Geometry: final body of the model. Coordinates: model frame, mm. A direction names the side the tool comes from. Give positions to 0.01 mm unless a question says otherwise; leave off trailing zeros.
1. Material intervals for line 1 along X through (y, z) = (-10.8, 421.85); line 2 along X through (y, z) = (11, 220) (3 decimals); line 3 along Y through (x, z) = (3, 393.5) (3 decimals), sorted ascending.
2. Access query for faces 1 (the face through (-2, -9.525, 332)), 2 (the face through (12.7, 0, 332)). Directions: +Z, -Z, +X, -X, +Y, -Y. A direction counts if a zero-diameter tool reaches every point of the face in a straight line with its end or side. Return the directions, or none.
3. First-contact query: P1, Ø12, axis at x = -1, y = -7.5, coming from the -Z side; P2, Ø4.5, axis at y = 2.38, z = 117.35, coming from the -X side (3 decimals); P3, Ø1, axis at y = -10, z = 199, coming from the -X side; P4, Ø4, axis at x = -2.38, z = 247.85, coming from the +Y side (3 decimals). Flat tips, straight axial feed; report the tip coordinate or a pass-through.
from build123d import *

# Parameters (mm, degrees)
BOSS_EXTRUDE1_DEPTH = 609.6
SKETCH3_W           = 655.2
SKETCH3_H           = 25.4
CUT_EXTRUDE2_DEPTH  = 30.48
SKETCH4_R           = 1.7
CUT_EXTRUDE4_DEPTH  = 611.137198198
SKETCH7_R           = 1.7
CUT_EXTRUDE6_DEPTH  = 611.137198198
CUT_EXTRUDE7_DEPTH  = 611.137198198
CUT_EXTRUDE8_DEPTH  = 611.137198198


with BuildPart() as part:
    # Sketch2 → Boss-Extrude1 (new, symmetric)
    with BuildSketch(Plane.XY):
        with BuildLine():
            Line((-12.7, -12.7), (12.7, -12.7))
            Line((12.7, -12.7), (12.7, 12.7))
            Line((12.7, 12.7), (11.1125, 12.7))
            ThreePointArc((11.1125, 12.7), (9.989967985, 12.235032015), (9.525, 11.1125))
            Line((9.525, 11.1125), (9.525, -6.35))
            ThreePointArc((9.525, -6.35), (8.59506403, -8.59506403), (6.35, -9.525))
            Line((6.35, -9.525), (-11.1125, -9.525))
            ThreePointArc((-11.1125, -9.525), (-12.235032015, -9.989967985), (-12.7, -11.1125))
            Line((-12.7, -11.1125), (-12.7, -12.7))
        make_face()
    extrude(amount=BOSS_EXTRUDE1_DEPTH, both=True)

    # Sketch3 → Cut-Extrude2 (cut)
    with BuildSketch(Plane(origin=(12.7, 0, 0), x_dir=(0, 0, -1), z_dir=(1, 0, 0))):
        with Locations((282, 0)):
            Rectangle(SKETCH3_W, SKETCH3_H)
    extrude(amount=-CUT_EXTRUDE2_DEPTH, mode=Mode.SUBTRACT)

    # Sketch4 → Cut-Extrude4 (cut, through all)
    with BuildSketch(Plane(origin=(0, -9.525, 0), x_dir=(1, 0, 0), z_dir=(0, 1, 0))):
        with Locations(Location((-2.38125, -552.35, 0), (0, 0, 180))):
            Circle(SKETCH4_R)
        with Locations(Location((-2.38125, -537.85, 0), (0, 0, 180))):
            Circle(SKETCH4_R)
        with Locations(Location((-2.38125, -523.35, 0), (0, 0, 180))):
            Circle(SKETCH4_R)
        with Locations(Location((-2.38125, -508.85, 0), (0, 0, 180))):
            Circle(SKETCH4_R)
        with Locations(Location((-2.38125, -494.35, 0), (0, 0, 180))):
            Circle(SKETCH4_R)
        with Locations(Location((-2.38125, -479.85, 0), (0, 0, 180))):
            Circle(SKETCH4_R)
        with Locations(Location((-2.38125, -465.35, 0), (0, 0, 180))):
            Circle(SKETCH4_R)
        with Locations(Location((-2.38125, -450.85, 0), (0, 0, 180))):
            Circle(SKETCH4_R)
        with Locations(Location((-2.38125, -436.35, 0), (0, 0, 180))):
            Circle(SKETCH4_R)
        with Locations(Location((-2.38125, -421.85, 0), (0, 0, 180))):
            Circle(SKETCH4_R)
        with Locations(Location((-2.38125, -407.35, 0), (0, 0, 180))):
            Circle(SKETCH4_R)
        with Locations(Location((-2.38125, -392.85, 0), (0, 0, 180))):
            Circle(SKETCH4_R)
        with Locations(Location((-2.38125, -378.35, 0), (0, 0, 180))):
            Circle(SKETCH4_R)
        with Locations(Location((-2.38125, -363.85, 0), (0, 0, 180))):
            Circle(SKETCH4_R)
        with Locations(Location((-2.38125, -349.35, 0), (0, 0, 180))):
            Circle(SKETCH4_R)
        with Locations(Location((-2.38125, -334.85, 0), (0, 0, 180))):
            Circle(SKETCH4_R)
        with Locations(Location((-2.38125, -320.35, 0), (0, 0, 180))):
            Circle(SKETCH4_R)
        with Locations(Location((-2.38125, -305.85, 0), (0, 0, 180))):
            Circle(SKETCH4_R)
        with Locations(Location((-2.38125, -291.35, 0), (0, 0, 180))):
            Circle(SKETCH4_R)
        with Locations(Location((-2.38125, -276.85, 0), (0, 0, 180))):
            Circle(SKETCH4_R)
        with Locations(Location((-2.38125, -262.35, 0), (0, 0, 180))):
            Circle(SKETCH4_R)
        with Locations(Location((-2.38125, -247.85, 0), (0, 0, 180))):
            Circle(SKETCH4_R)
        with Locations(Location((-2.38125, -233.35, 0), (0, 0, 180))):
            Circle(SKETCH4_R)
        with Locations(Location((-2.38125, -218.85, 0), (0, 0, 180))):
            Circle(SKETCH4_R)
        with Locations(Location((-2.38125, -204.35, 0), (0, 0, 180))):
            Circle(SKETCH4_R)
        with Locations(Location((-2.38125, -189.85, 0), (0, 0, 180))):
            Circle(SKETCH4_R)
        with Locations(Location((-2.38125, -175.35, 0), (0, 0, 180))):
            Circle(SKETCH4_R)
        with Locations(Location((-2.38125, -160.85, 0), (0, 0, 180))):
            Circle(SKETCH4_R)
        with Locations(Location((-2.38125, -146.35, 0), (0, 0, 180))):
            Circle(SKETCH4_R)
        with Locations(Location((-2.38125, -131.85, 0), (0, 0, 180))):
            Circle(SKETCH4_R)
        with Locations(Location((-2.38125, -117.35, 0), (0, 0, 180))):
            Circle(SKETCH4_R)
        with Locations(Location((-2.38125, -102.85, 0), (0, 0, 180))):
            Circle(SKETCH4_R)
    extrude(amount=-CUT_EXTRUDE4_DEPTH, mode=Mode.SUBTRACT)

    # Sketch7 → Cut-Extrude6 (cut, through all)
    with BuildSketch(Plane.ZY.offset(-9.525)):
        with Locations(Location((552.35, 2.38125, 0), (0, 0, 270))):
            Circle(SKETCH7_R)
        with Locations(Location((537.85, 2.38125, 0), (0, 0, 270))):
            Circle(SKETCH7_R)
        with Locations(Location((523.35, 2.38125, 0), (0, 0, 270))):
            Circle(SKETCH7_R)
        with Locations(Location((508.85, 2.38125, 0), (0, 0, 270))):
            Circle(SKETCH7_R)
        with Locations(Location((494.35, 2.38125, 0), (0, 0, 270))):
            Circle(SKETCH7_R)
        with Locations(Location((479.85, 2.38125, 0), (0, 0, 270))):
            Circle(SKETCH7_R)
        with Locations(Location((465.35, 2.38125, 0), (0, 0, 270))):
            Circle(SKETCH7_R)
        with Locations(Location((450.85, 2.38125, 0), (0, 0, 270))):
            Circle(SKETCH7_R)
        with Locations(Location((436.35, 2.38125, 0), (0, 0, 270))):
            Circle(SKETCH7_R)
        with Locations(Location((421.85, 2.38125, 0), (0, 0, 270))):
            Circle(SKETCH7_R)
        with Locations(Location((407.35, 2.38125, 0), (0, 0, 270))):
            Circle(SKETCH7_R)
        with Locations(Location((392.85, 2.38125, 0), (0, 0, 270))):
            Circle(SKETCH7_R)
        with Locations(Location((378.35, 2.38125, 0), (0, 0, 270))):
            Circle(SKETCH7_R)
        with Locations(Location((363.85, 2.38125, 0), (0, 0, 270))):
            Circle(SKETCH7_R)
        with Locations(Location((349.35, 2.38125, 0), (0, 0, 270))):
            Circle(SKETCH7_R)
        with Locations(Location((334.85, 2.38125, 0), (0, 0, 270))):
            Circle(SKETCH7_R)
        with Locations(Location((320.35, 2.38125, 0), (0, 0, 270))):
            Circle(SKETCH7_R)
        with Locations(Location((305.85, 2.38125, 0), (0, 0, 270))):
            Circle(SKETCH7_R)
        with Locations(Location((291.35, 2.38125, 0), (0, 0, 270))):
            Circle(SKETCH7_R)
        with Locations(Location((276.85, 2.38125, 0), (0, 0, 270))):
            Circle(SKETCH7_R)
        with Locations(Location((262.35, 2.38125, 0), (0, 0, 270))):
            Circle(SKETCH7_R)
        with Locations(Location((247.85, 2.38125, 0), (0, 0, 270))):
            Circle(SKETCH7_R)
        with Locations(Location((233.35, 2.38125, 0), (0, 0, 270))):
            Circle(SKETCH7_R)
        with Locations(Location((218.85, 2.38125, 0), (0, 0, 270))):
            Circle(SKETCH7_R)
        with Locations(Location((204.35, 2.38125, 0), (0, 0, 270))):
            Circle(SKETCH7_R)
        with Locations(Location((189.85, 2.38125, 0), (0, 0, 270))):
            Circle(SKETCH7_R)
        with Locations(Location((175.35, 2.38125, 0), (0, 0, 270))):
            Circle(SKETCH7_R)
        with Locations(Location((160.85, 2.38125, 0), (0, 0, 270))):
            Circle(SKETCH7_R)
        with Locations(Location((146.35, 2.38125, 0), (0, 0, 270))):
            Circle(SKETCH7_R)
        with Locations(Location((131.85, 2.38125, 0), (0, 0, 270))):
            Circle(SKETCH7_R)
        with Locations(Location((117.35, 2.38125, 0), (0, 0, 270))):
            Circle(SKETCH7_R)
        with Locations(Location((102.85, 2.38125, 0), (0, 0, 270))):
            Circle(SKETCH7_R)
    extrude(amount=-CUT_EXTRUDE6_DEPTH, mode=Mode.SUBTRACT)

    # Sketch8 → Cut-Extrude7 (cut, through all)
    with BuildSketch(Plane.ZY.offset(-9.525)):
        with BuildLine():
            Line((49.3305, 4.0825), (52.7305, 4.0825))
            ThreePointArc((52.7305, 4.0825), (54.4305, 2.3825), (52.7305, 0.6825))
            Line((52.7305, 0.6825), (49.3305, 0.6825))
            ThreePointArc((49.3305, 0.6825), (47.6305, 2.3825), (49.3305, 4.0825))
        make_face()
        with BuildLine():
            Line((78.0325, 4.0825), (81.4325, 4.0825))
            ThreePointArc((81.4325, 4.0825), (83.1325, 2.3825), (81.4325, 0.6825))
            Line((81.4325, 0.6825), (78.0325, 0.6825))
            ThreePointArc((78.0325, 0.6825), (76.3325, 2.3825), (78.0325, 4.0825))
        make_face()
        with BuildLine():
            Line((573.7675, 4.0825), (577.1675, 4.0825))
            ThreePointArc((577.1675, 4.0825), (578.8675, 2.3825), (577.1675, 0.6825))
            Line((577.1675, 0.6825), (573.7675, 0.6825))
            ThreePointArc((573.7675, 0.6825), (572.0675, 2.3825), (573.7675, 4.0825))
        make_face()
        with BuildLine():
            Line((602.4695, 4.0825), (605.8695, 4.0825))
            ThreePointArc((605.8695, 4.0825), (607.5695, 2.3825), (605.8695, 0.6825))
            Line((605.8695, 0.6825), (602.4695, 0.6825))
            ThreePointArc((602.4695, 0.6825), (600.7695, 2.3825), (602.4695, 4.0825))
        make_face()
    extrude(amount=-CUT_EXTRUDE7_DEPTH, mode=Mode.SUBTRACT)

    # Sketch9 → Cut-Extrude8 (cut, through all)
    with BuildSketch(Plane(origin=(0, -9.525, 0), x_dir=(1, 0, 0), z_dir=(0, 1, 0))):
        with BuildLine():
            Line((-4.0825, -605.8695), (-4.0825, -602.4695))
            ThreePointArc((-4.0825, -602.4695), (-2.3825, -600.7695), (-0.6825, -602.4695))
            Line((-0.6825, -602.4695), (-0.6825, -605.8695))
            ThreePointArc((-0.6825, -605.8695), (-2.3825, -607.5695), (-4.0825, -605.8695))
        make_face()
        with BuildLine():
            Line((-4.0825, -577.1675), (-4.0825, -573.7675))
            ThreePointArc((-4.0825, -573.7675), (-2.3825, -572.0675), (-0.6825, -573.7675))
            Line((-0.6825, -573.7675), (-0.6825, -577.1675))
            ThreePointArc((-0.6825, -577.1675), (-2.3825, -578.8675), (-4.0825, -577.1675))
        make_face()
        with BuildLine():
            Line((-4.0825, -81.4325), (-4.0825, -78.0325))
            ThreePointArc((-4.0825, -78.0325), (-2.3825, -76.3325), (-0.6825, -78.0325))
            Line((-0.6825, -78.0325), (-0.6825, -81.4325))
            ThreePointArc((-0.6825, -81.4325), (-2.3825, -83.1325), (-4.0825, -81.4325))
        make_face()
        with BuildLine():
            Line((-4.0825, -52.7305), (-4.0825, -49.3305))
            ThreePointArc((-4.0825, -49.3305), (-2.3825, -47.6305), (-0.6825, -49.3305))
            Line((-0.6825, -49.3305), (-0.6825, -52.7305))
            ThreePointArc((-0.6825, -52.7305), (-2.3825, -54.4305), (-4.0825, -52.7305))
        make_face()
    extrude(amount=-CUT_EXTRUDE8_DEPTH, mode=Mode.SUBTRACT)


solid = part.part
Answers below:
1. line 1: x = -12.67 to -4.08, -0.68 to 12.7
1. line 2: x = 9.525 to 12.7
1. line 3: y = -12.7 to -9.525
2. face 1: +Z, -Z, -X, +Y
2. face 2: +Z, -Z, +X, +Y, -Y
3. P1: stops at z = 45.6
3. P2: stops at x = 9.525
3. P3: stops at x = -12.58
3. P4: stops at y = -9.525
